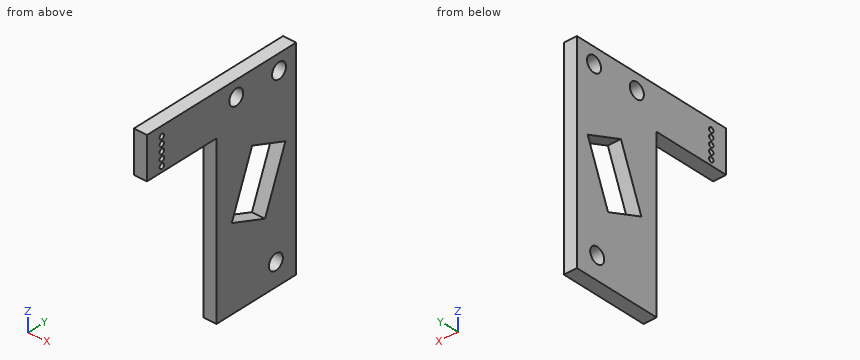
from build123d import *

# Parameters (mm, degrees)
SKETCH1_R           = 2.38125
SKETCH1_R_2         = 0.75
BOSS_EXTRUDE1_DEPTH = 2


with BuildPart() as part:
    # Sketch1 → Boss-Extrude1 (new, symmetric)
    with BuildSketch(Plane(origin=(0, 0, 0), x_dir=(0, 0, -1), z_dir=(1, 0, 0))):
        Polygon((6.909587278, 6.909587278), (-56.590412722, 6.909587278), (-56.590412722, -43.890412722), (-43.890412722, -43.890412722), (-43.890412722, -20.222057583), (6.909587278, -20.222057583), align=None)
        Circle(SKETCH1_R, mode=Mode.SUBTRACT)
        with Locations((-45.552958224, -38.810412722)):
            Circle(SKETCH1_R_2, mode=Mode.SUBTRACT)
        with Locations((-47.584958224, -38.810412722)):
            Circle(SKETCH1_R_2, mode=Mode.SUBTRACT)
        with Locations((-49.616958224, -38.810412722)):
            Circle(SKETCH1_R_2, mode=Mode.SUBTRACT)
        with Locations((-51.648958224, -38.810412722)):
            Circle(SKETCH1_R_2, mode=Mode.SUBTRACT)
        with Locations((-51.818112153, -13.484149416)):
            Circle(SKETCH1_R, mode=Mode.SUBTRACT)
        with Locations((-51.818112153, 1.079375692)):
            Circle(SKETCH1_R, mode=Mode.SUBTRACT)
        with Locations((-53.680958224, -38.810412722)):
            Circle(SKETCH1_R_2, mode=Mode.SUBTRACT)
        Polygon((-31.413305249, 3.250726227), (-13.673130295, -3.691081364), (-18.105513832, -15.018283734), (-35.845688785, -8.076476144), align=None, mode=Mode.SUBTRACT)
    extrude(amount=BOSS_EXTRUDE1_DEPTH, both=True)


solid = part.part
Verification items for the finished model (mm, model axes). Coordinates: 2 decimals unless noted, no trailing zeros. Order: outer loops, then holes, each group sorted by start corner. A loop starts at its lowest first (then second) coordinate and runs counter-clockwise, first axis right, second up. Notation, with made-up numbers: M 9.5,65 L 68.5,65 A18 ccw 68.5,92 Z; hole C -10,-23.5 d3. An arc over 180 degrees is marked long. Write each question's results on one line, items separated by ' | '.
1) Section check A-A on z = 0. Record the cut outline in (x, y), plus the area to 3 significant figures.
Solved:
outline: M -2,-20.22 L 2,-20.22 L 2,-2.38 L -2,-2.38 Z; M -2,2.38 L 2,2.38 L 2,6.91 L -2,6.91 Z | area: 89.5 mm²
2) Scan lines: line 1 along Y through (x, z) = (-0.1, 45.5); line 2 along Z through (x, y) = (1, -39); line 3 along Y through (x, z) = (-1.1, 8). Record each from-to range of solid material in increasing order. Write a range as [from, to].
Solved:
line 1: y = [-43.89, -39.56], [-38.06, 6.91] | line 2: z = [43.89, 44.83], [46.28, 46.86], [48.31, 48.89], [50.34, 50.92], [52.37, 52.96], [54.41, 56.59] | line 3: y = [-20.22, 6.91]
3) Section check B-B on y = -5. Record the cut outline in (x, z).
Solved:
outline: M -2,-6.91 L 2,-6.91 L 2,14.19 L -2,14.19 Z; M -2,34.64 L 2,34.64 L 2,56.59 L -2,56.59 Z
4) Gauge pin test, flat end, axial feed: pin 1 Ø1.4 at (y, z) = (-38.81, 45.55) entering from -X. Record the tip position at first contact, or that the pin passes through.
Solved:
pin 1: passes through
5) Section check D-D on z = 43. Record the cut outline in (x, y), plus the area to 3 significant figures.
Solved:
outline: M -2,-20.22 L 2,-20.22 L 2,6.91 L -2,6.91 Z | area: 109 mm²
6) Section check C-C on x = -0.05. Give the number of separate pieces and of enclosed holes in the cut face, plus the area to 3 significant figures.
Solved:
separate pieces: 1 | enclosed holes: 9 | area: 1,730 mm²
